Geometry check sheet. Reference: the model listing, model coordinates, mm. A direction names the side the tool comes from. Give positions to 0.01 mm unless a question says otherwise; leave off trailing zeros. Write each loop counter-clockwise with the first axis right and the second up, starting at its lowest first coordinate (ties: lowest second). Pieces come first, ordered by that corner, then holes. Notation, with made-up numbers: (89, -24) -> (102, -24) arc R28 ccw to (102, 11) -> close; hole circle Ø2 at (-35, -26.5). An arc over 180 degrees is marked (long way). One line per item, written item: value.
from build123d import *

# Parameters (mm, degrees)
ESQUISSE1_W             = 200
ESQUISSE1_H             = 300
BOSS_EXTRU_1_DEPTH      = 80
COQUE1_T                = -4
ESQUISSE3_W             = 196.2
ESQUISSE3_H             = 296.2
ENL_V_MAT_EXTRU_2_DEPTH = 4.1
ESQUISSE4_R             = 9
BOSS_EXTRU_2_DEPTH      = 67.9
ESQUISSE5_R             = 2.5
ENL_V_MAT_EXTRU_3_DEPTH = 30
ESQUISSE4_4_R           = 9
BOSS_EXTRU_3_DEPTH      = 15
ESQUISSE6_R             = 2.5
ENL_V_MAT_EXTRU_6_DEPTH = 10
ESQUISSE8_R             = 9
BOSS_EXTRU_5_DEPTH      = 68
ESQUISSE9_R             = 2.5
ENL_V_MAT_EXTRU_8_DEPTH = 30


with BuildPart() as part:
    # Esquisse1 → Boss.-Extru.1 (new body)
    with BuildSketch(Plane.XY):
        with Locations((43.373964051, -118.711656442)):
            Rectangle(ESQUISSE1_W, ESQUISSE1_H)
    extrude(amount=BOSS_EXTRU_1_DEPTH)

    # Coque1
    coque1_openings = [part.faces().sort_by_distance(p)[0] for p in [
        (43.373964051, -118.711656442, 0),
    ]]
    offset(amount=COQUE1_T, openings=coque1_openings, kind=Kind.INTERSECTION)

    # Esquisse3 → Enl_v. mat.-Extru.2 (cut)
    with BuildSketch(Plane(origin=(0, 0, 0), x_dir=(-1, 0, 0), z_dir=(0, 0, -1))):
        with Locations((-43.373964051, -118.711656442)):
            Rectangle(ESQUISSE3_W, ESQUISSE3_H)
    extrude(amount=-ENL_V_MAT_EXTRU_2_DEPTH, mode=Mode.SUBTRACT)

    # Esquisse4 → Boss.-Extru.2 (add)
    with BuildSketch(Plane(origin=(0, 0, 76), x_dir=(-1, 0, 0), z_dir=(0, 0, -1))):
        with Locations(Location((-119.373964051, 7.288343558, 0), (0, 0, 180))):
            Circle(ESQUISSE4_R)
    extrude(amount=BOSS_EXTRU_2_DEPTH)

    # Esquisse5 → Enl_v. mat.-Extru.3 (cut)
    with BuildSketch(Plane(origin=(0, 0, 8.1), x_dir=(-1, 0, 0), z_dir=(0, 0, -1))):
        with Locations((-119.373964051, 7.288343558)):
            Circle(ESQUISSE5_R)
    extrude(amount=-ENL_V_MAT_EXTRU_3_DEPTH, mode=Mode.SUBTRACT)

    # Esquisse4_4 → Boss.-Extru.3 (add)
    with BuildSketch(Plane(origin=(0, 0, 76), x_dir=(-1, 0, 0), z_dir=(0, 0, -1))):
        with BuildLine():
            Line((-89.373964051, -53.711656442), (-89.373964051, -62.711656442))
            Line((-89.373964051, -62.711656442), (-98.373964051, -62.711656442))
            ThreePointArc((-98.373964051, -62.711656442), (-89.373964051, -71.711656442), (-80.373964051, -62.711656442))
            ThreePointArc((-80.373964051, -62.711656442), (-83.010003021, -56.347695411), (-89.373964051, -53.711656442))
        make_face()
        with BuildLine():
            Line((-98.373964051, -62.711656442), (-89.373964051, -62.711656442))
            Line((-89.373964051, -62.711656442), (-89.373964051, -53.711656442))
            ThreePointArc((-89.373964051, -53.711656442), (-95.737925082, -56.347695411), (-98.373964051, -62.711656442))
        make_face()
        with BuildLine():
            Line((-89.373964051, -53.711656442), (-89.373964051, -62.711656442))
            Line((-89.373964051, -62.711656442), (-98.373964051, -62.711656442))
            ThreePointArc((-98.373964051, -62.711656442), (-89.373964051, -71.711656442), (-80.373964051, -62.711656442))
            ThreePointArc((-80.373964051, -62.711656442), (-83.010003021, -56.347695411), (-89.373964051, -53.711656442))
        make_face()
        with BuildLine():
            Line((-98.373964051, -62.711656442), (-89.373964051, -62.711656442))
            Line((-89.373964051, -62.711656442), (-89.373964051, -53.711656442))
            ThreePointArc((-89.373964051, -53.711656442), (-95.737925082, -56.347695411), (-98.373964051, -62.711656442))
        make_face()
        with BuildLine():
            Line((2.626035949, -183.711656442), (2.626035949, -174.711656442))
            Line((2.626035949, -174.711656442), (11.626035949, -174.711656442))
            ThreePointArc((11.626035949, -174.711656442), (-3.737925082, -168.347695411), (2.626035949, -183.711656442))
        make_face()
        with BuildLine():
            Line((11.626035949, -174.711656442), (2.626035949, -174.711656442))
            Line((2.626035949, -174.711656442), (2.626035949, -183.711656442))
            ThreePointArc((2.626035949, -183.711656442), (8.989996979, -181.075617472), (11.626035949, -174.711656442))
        make_face()
        with BuildLine():
            Line((2.626035949, -183.711656442), (2.626035949, -174.711656442))
            Line((2.626035949, -174.711656442), (11.626035949, -174.711656442))
            ThreePointArc((11.626035949, -174.711656442), (-3.737925082, -168.347695411), (2.626035949, -183.711656442))
        make_face()
        with BuildLine():
            Line((11.626035949, -174.711656442), (2.626035949, -174.711656442))
            Line((2.626035949, -174.711656442), (2.626035949, -183.711656442))
            ThreePointArc((2.626035949, -183.711656442), (8.989996979, -181.075617472), (11.626035949, -174.711656442))
        make_face()
        with Locations(Location((2.626035949, -62.711656442, 0), (0, 0, 180))):
            Circle(ESQUISSE4_4_R)
        with Locations(Location((-89.373964051, -174.711656442, 0), (0, 0, 180))):
            Circle(ESQUISSE4_4_R)
    extrude(amount=BOSS_EXTRU_3_DEPTH)

    # Esquisse6 → Enl_v. mat.-Extru.6 (cut)
    with BuildSketch(Plane(origin=(0, 0, 61), x_dir=(-1, 0, 0), z_dir=(0, 0, -1))):
        with Locations((-89.373964051, -62.711656442)):
            Circle(ESQUISSE6_R)
        with Locations((2.626035949, -62.711656442)):
            Circle(ESQUISSE6_R)
        with Locations((-89.373964051, -174.711656442)):
            Circle(ESQUISSE6_R)
        with Locations((2.626035949, -174.711656442)):
            Circle(ESQUISSE6_R)
    extrude(amount=-ENL_V_MAT_EXTRU_6_DEPTH, mode=Mode.SUBTRACT)

    # Esquisse8 → Boss.-Extru.5 (add)
    with BuildSketch(Plane(origin=(0, 0, 76), x_dir=(-1, 0, 0), z_dir=(0, 0, -1))):
        with BuildLine():
            Line((32.626035949, 16.288343558), (32.626035949, 7.288343558))
            Line((32.626035949, 7.288343558), (41.626035949, 7.288343558))
            ThreePointArc((41.626035949, 7.288343558), (38.989996979, 13.652304589), (32.626035949, 16.288343558))
        make_face()
        with BuildLine():
            Line((41.626035949, 7.288343558), (32.626035949, 7.288343558))
            Line((32.626035949, 7.288343558), (32.626035949, 16.288343558))
            ThreePointArc((32.626035949, 16.288343558), (26.262074918, 0.924382528), (41.626035949, 7.288343558))
        make_face()
        with BuildLine():
            Line((32.626035949, 16.288343558), (32.626035949, 7.288343558))
            Line((32.626035949, 7.288343558), (41.626035949, 7.288343558))
            ThreePointArc((41.626035949, 7.288343558), (38.989996979, 13.652304589), (32.626035949, 16.288343558))
        make_face()
        with BuildLine():
            Line((41.626035949, 7.288343558), (32.626035949, 7.288343558))
            Line((32.626035949, 7.288343558), (32.626035949, 16.288343558))
            ThreePointArc((32.626035949, 16.288343558), (26.262074918, 0.924382528), (41.626035949, 7.288343558))
        make_face()
        with BuildLine():
            Line((32.626035949, -253.711656442), (32.626035949, -244.711656442))
            Line((32.626035949, -244.711656442), (41.626035949, -244.711656442))
            ThreePointArc((41.626035949, -244.711656442), (26.262074918, -238.347695411), (32.626035949, -253.711656442))
        make_face()
        with BuildLine():
            Line((41.626035949, -244.711656442), (32.626035949, -244.711656442))
            Line((32.626035949, -244.711656442), (32.626035949, -253.711656442))
            ThreePointArc((32.626035949, -253.711656442), (38.989996979, -251.075617472), (41.626035949, -244.711656442))
        make_face()
        with BuildLine():
            Line((32.626035949, -253.711656442), (32.626035949, -244.711656442))
            Line((32.626035949, -244.711656442), (41.626035949, -244.711656442))
            ThreePointArc((41.626035949, -244.711656442), (26.262074918, -238.347695411), (32.626035949, -253.711656442))
        make_face()
        with BuildLine():
            Line((41.626035949, -244.711656442), (32.626035949, -244.711656442))
            Line((32.626035949, -244.711656442), (32.626035949, -253.711656442))
            ThreePointArc((32.626035949, -253.711656442), (38.989996979, -251.075617472), (41.626035949, -244.711656442))
        make_face()
        with Locations(Location((-119.373964051, -244.711656442, 0), (0, 0, 180))):
            Circle(ESQUISSE8_R)
    extrude(amount=BOSS_EXTRU_5_DEPTH)

    # Esquisse9 → Enl_v. mat.-Extru.8 (cut)
    with BuildSketch(Plane(origin=(0, 0, 8), x_dir=(-1, 0, 0), z_dir=(0, 0, -1))):
        with Locations((32.626035949, 7.288343558)):
            Circle(ESQUISSE9_R)
        with Locations((32.626035949, -244.711656442)):
            Circle(ESQUISSE9_R)
        with Locations((-119.373964051, -244.711656442)):
            Circle(ESQUISSE9_R)
    extrude(amount=-ENL_V_MAT_EXTRU_8_DEPTH, mode=Mode.SUBTRACT)


solid = part.part
1) Depth check by flat-ended pin: pin 1 Ø14.5 at (x, y) = (-29, 5) entering from -Z; pin 2 Ø4 at (x, y) = (90.5, -62.5) entering from -Z; pin 3 Ø2.5 at (x, y) = (-32.5, 8) entering from -Z. Enter the tip coordinate at first touch or a pass-through.
Verdict:
pin 1: z = 8
pin 2: z = 61
pin 3: z = 38
2) Mould release check, pull along Y, two halves, no side actions. Record for faces 3 (the flat face through (42, 31.288, 39)), 4 (the flat face through (-0.75, -60.84, 61)), 5 (the flat face through (121.25, -242.84, 8)), 6 (the flat face through (-56.626, -121, 39)): released by +Y, released by -Y, zero draft, split by the parting line, or undercut.
Verdict:
face 3: released by +Y
face 4: undercut
face 5: undercut
face 6: zero draft
3) Sectioned sample at C-C on y = -157. Record the cut outline in (x, z).
Verdict:
outline: (-56.63, 0) -> (-54.73, 0) -> (-54.73, 4.1) -> (-52.63, 4.1) -> (-52.63, 76) -> (139.37, 76) -> (139.37, 4.1) -> (141.47, 4.1) -> (141.47, 0) -> (143.37, 0) -> (143.37, 80) -> (-56.63, 80) -> close
4) Sectioned sample at B-B on z = 46.5. Record the cut outline in (x, y).
Verdict:
outline: (-56.63, -268.71) -> (143.37, -268.71) -> (143.37, 31.29) -> (-56.63, 31.29) -> close; circle Ø18 at (-32.63, -244.71); circle Ø18 at (-32.63, 7.29); circle Ø18 at (119.37, -244.71); circle Ø18 at (119.37, 7.29); hole (-52.63, -264.71) -> (139.37, -264.71) -> (139.37, 27.29) -> (-52.63, 27.29) -> close
5) Sectioned sample at A-A on z = 11.5. Give the number of separate pieces and of enclosed holes in the cut face, plus the area to 3 significant figures.
Verdict:
separate pieces: 5
enclosed holes: 5
area: 4,880 mm^2
6) Scan lines: probe 1 along X at (y, z) = (-18, 43); probe 2 along Y at (x, z) = (97, 27.5); probe 3 along Y at (x, z) = (-31.5, 29). Record each from-to range of solid material in increasing order.
Verdict:
probe 1: -56.63 to -52.63, 139.37 to 143.37
probe 2: -268.71 to -264.71, 27.29 to 31.29
probe 3: -268.71 to -264.71, -253.64 to -246.94, -242.48 to -235.78, -1.64 to 5.06, 9.52 to 16.22, 27.29 to 31.29
7) Tool access check on faces 1 (the flat face through (42, -268.712, 39)), 2 (the flat face through (-35, 5, 8)). Record the directions out of +Z, -Z, +X, -X, +Y, -Y that give a thin tool (end or side, any length) a straight path to the whole face; none if there is none.
Verdict:
face 1: +Z, -Z, +X, -X, -Y
face 2: -Z
8) Sectioned sample at D-D on x = 17. Record the cut outline in (y, z).
Verdict:
outline: (-268.71, 0) -> (-266.81, 0) -> (-266.81, 4.1) -> (-264.71, 4.1) -> (-264.71, 76) -> (27.29, 76) -> (27.29, 4.1) -> (29.39, 4.1) -> (29.39, 0) -> (31.29, 0) -> (31.29, 80) -> (-268.71, 80) -> close
